Design review of the part shown in the three views and the two pictorial views. Dimensions are in mm from the part's minimum x, y and z. Round coordinates to 2 decimals unless told otherwise and drop trailing zeros. Loops run counter-clockwise (first coordinate to the right, second up) from the corner with the lowest first, then second, coordinate; pieces in that order, holes last. Notation, with made-up numbers: (-16, 38) -> (19, 38) arc R20 cw to (19, 45) -> close; hole circle Ø7 at (64.25, 7). An arc over 180 degrees is marked (long way). Write each question's results on one line, items separated by ' | '. Start each with the question number.
Item 1: Clearance check with flat-ended pins moving along their axes: pin 1 Ø1.5 at (x, z) = (11.5, 26) entering from -Y; pin 2 Ø1 at (x, z) = (4, 20.5) entering from -Y; pin 3 Ø1.5 at (x, y) = (12.5, 1.5) entering from +Z; pin 4 Ø1.5 at (y, z) = (1, 2) entering from +X. State where each tip first meets the part, or that it passes through.
Item 2: We need section A-A (z = 20). Give the boundary of the cut face in (x, y), and give its area (3 significant figures).
Item 3: For L1, parallel to X at y = 2.45, z = 23; L2, parallel to Z at x = 13, y = 1; L3, parallel to X at y = 2.2, z = 2.75, list the stretches that pass through material, from the lowest coordinate up. Write a range as from..to.
Item 4: We need section C-C (x = 12.25). Give the boundary of the cut face in (y, z).
Item 5: We need section B-B (y = 1.2). Give the boundary of the cut face in (x, z), and give its area (3 significant figures).
Item 6: We need section D-D (z = 4). Give the boundary of the cut face in (x, y), and give its area (3 significant figures).
Item 7: Mouldability with a two-part tool opening along X and no side actions: class the marked faces 1 and 2 as pulls with the +X half, pulls with the -X half, needs draft (parallel to the pull), parting line crosses it, or undercut.
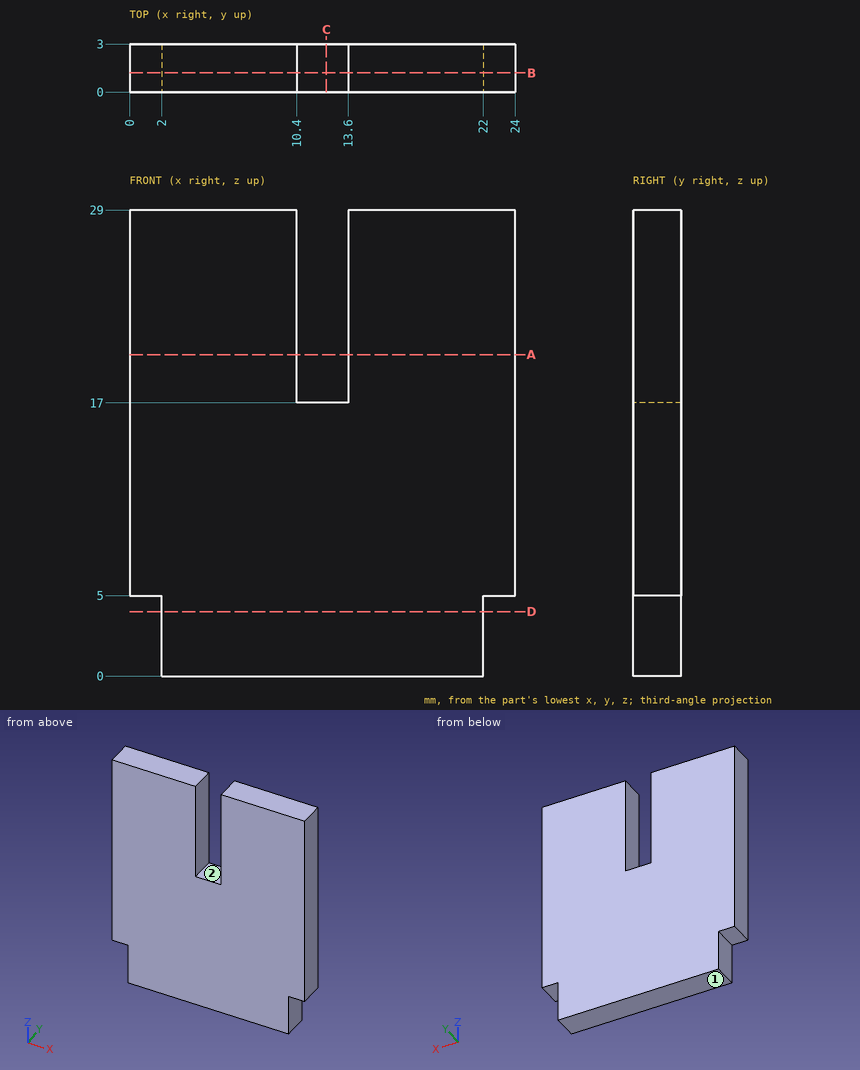
Here are the results:
1) pin 1: passes through | pin 2: stops at y = 0 | pin 3: stops at z = 17 | pin 4: stops at x = 22
2) outline: (0, 0) -> (10.4, 0) -> (10.4, 3) -> (0, 3) -> close; (13.6, 0) -> (24, 0) -> (24, 3) -> (13.6, 3) -> close | area: 62.4 mm2
3) L1: x = 0..10.4, 13.6..24 | L2: z = 0..17 | L3: x = 2..22
4) outline: (0, 0) -> (3, 0) -> (3, 17) -> (0, 17) -> close
5) outline: (0, 5) -> (2, 5) -> (2, 0) -> (22, 0) -> (22, 5) -> (24, 5) -> (24, 29) -> (13.6, 29) -> (13.6, 17) -> (10.4, 17) -> (10.4, 29) -> (0, 29) -> close | area: 638 mm2
6) outline: (2, 0) -> (22, 0) -> (22, 3) -> (2, 3) -> close | area: 60.0 mm2
7) face 1: needs draft | face 2: undercut
